```python
from build123d import *

# Parameters (mm, degrees)
SKETCH1_W           = 101.6
SKETCH1_H           = 76.2
BOSS_EXTRUDE1_DEPTH = 9.525
SKETCH2_W           = 4.7625
SKETCH2_H           = 76.2
BOSS_EXTRUDE2_DEPTH = 44.45
SKETCH3_W           = 76.2
SKETCH3_H           = 4.7625
BOSS_EXTRUDE3_DEPTH = 7.9375
BOSS_EXTRUDE4_DEPTH = 101.6
CUT_EXTRUDE1_DEPTH  = 142.599304818


with BuildPart() as part:
    # Sketch1 → Boss-Extrude1 (new body)
    with BuildSketch(Plane(origin=(0, 0, 0), x_dir=(1, 0, 0), z_dir=(0, 1, 0))):
        with Locations((50.8, 38.1)):
            Rectangle(SKETCH1_W, SKETCH1_H)
    extrude(amount=BOSS_EXTRUDE1_DEPTH)

    # Sketch2 → Boss-Extrude2 (add)
    with BuildSketch(Plane(origin=(0, 9.525, 0), x_dir=(1, 0, 0), z_dir=(0, 1, 0))):
        with Locations((29.36875, 38.1)):
            Rectangle(SKETCH2_W, SKETCH2_H)
    boss_extrude2 = extrude(amount=BOSS_EXTRUDE2_DEPTH)

    # Sketch3 → Boss-Extrude3 (add)
    with BuildSketch(Plane(origin=(31.75, 0, 0), x_dir=(0, 0, -1), z_dir=(1, 0, 0))):
        with Locations((38.1, 51.59375)):
            Rectangle(SKETCH3_W, SKETCH3_H)
    boss_extrude3 = extrude(amount=BOSS_EXTRUDE3_DEPTH)

    # Mirror1: Boss-Extrude2, Boss-Extrude3 across plane
    add(boss_extrude2.mirror(Plane(origin=(50.8, 0, 0), x_dir=(0, 0, 1), z_dir=(1, 0, 0))))
    add(boss_extrude3.mirror(Plane(origin=(50.8, 0, 0), x_dir=(0, 0, 1), z_dir=(1, 0, 0))))

    # Sketch7 → Boss-Extrude4 (add)
    with BuildSketch(Plane(origin=(101.6, 0, 0), x_dir=(0, 0, -1), z_dir=(1, 0, 0))):
        Polygon((76.2, 3.175), (76.2, 6.35), (82.55, 8.03294256), (82.55, 1.682230673), align=None)
    extrude(amount=-BOSS_EXTRUDE4_DEPTH)

    # Sketch9 → Cut-Extrude1 (cut, through all)
    with BuildSketch(Plane(origin=(101.6, 0, 0), x_dir=(0, 0, -1), z_dir=(1, 0, 0))):
        Polygon((0, 2.921), (0, 6.604), (6.35, 8.1915), (6.35, 1.3335), align=None)
    extrude(amount=-CUT_EXTRUDE1_DEPTH, mode=Mode.SUBTRACT)


solid = part.part
```
Could you check a few things on this model? Use its own coordinates, in mm. A direction names the side the tool comes from. Give positions to 0.01 mm unless a question says otherwise; leave off trailing zeros. Order: outer loops, then holes, each group sorted by start corner. A loop starts at its lowest first (then second) coordinate and runs counter-clockwise, first axis right, second up.
Q1. If I drill on line 1 along X through (y, z) = (15.5, -10.5); line 2 along Y through (x, z) = (35, -28.5) (1 decimal); line 3 along Y through (x, z) = (17, -51) (3 decimals), over which ranges is the centre line in solid material (lowest first)?
Q2. We'd pull the mould along Z, two halves only. Please class faces 6 (the flat face through (51.51, 2.42, -79.42)), 7 (the flat face through (52, 5, -82.55)), 8 (the flat face through (39.688, 52, -38)): +Z half, -Z half, draft (parallel to the pull), parting line (faces both ways), or undercut.
Q3. For faces 1 (the flat face through (52, 5, -6.35)), 2 (the flat face through (31.75, 29, -38)), 3 (the flat face through (88, 9.525, -39)), 4 (the flat face through (52, 2, -76.2)), 5 (the flat face through (51, 9, -76.2)), which set-ups out of +Z, -Z, +X, -X, +Y, -Y let a thin tool reach every point of the face, with its end or its side?
Q4. Suppose I cut it at A-A, the plane y = 38. Write out the boundary of the cut face in (x, z).
Q5. I'm going to push flat-ended pins straight in: P1, Ø13.5, axis at y = 23.5, z = -48.5, coming from the +X side; P2, Ø22, axis at y = 32, z = -20.5, coming from the -X side; P3, Ø24, axis at x = 73.5, y = 23.5, coming from the -Z side. Where does each tip first touch, or does it pass through?
Solution:
1. line 1: x = 26.99 to 31.75, 69.85 to 74.61
1. line 2: y = 0 to 9.5, 49.2 to 54
1. line 3: y = 0 to 9.525
2. face 6: undercut
2. face 7: -Z half
2. face 8: draft
3. face 1: +X, -X
3. face 2: +Z, -Z
3. face 3: +Z, -Z, +X, +Y
3. face 4: +X, -X, -Y
3. face 5: +X, -X, +Y
4. outline: (26.99, -76.2) - (31.75, -76.2) - (31.75, 0) - (26.99, 0) - close; (69.85, -76.2) - (74.61, -76.2) - (74.61, 0) - (69.85, 0) - close
5. P1: stops at x = 74.61
5. P2: stops at x = 26.99
5. P3: stops at z = -76.2
